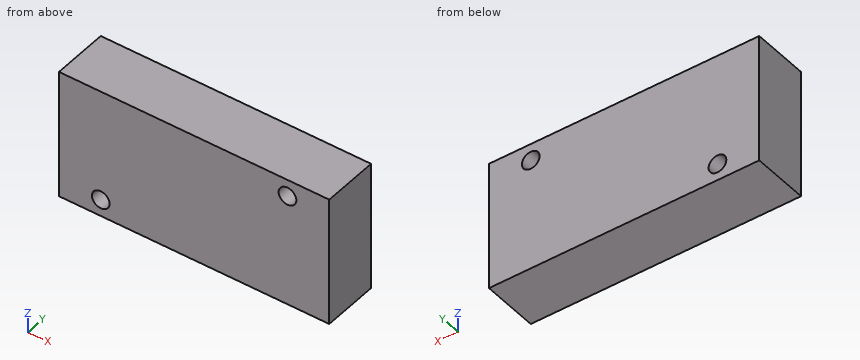
Autodesk Inventor part; units mm, degrees
ref_plane "YZ Plane" through (0, 0, 0) normal (1, 0, 0) x (0, 1, 0)
ref_plane "XZ Plane" through (0, 0, 0) normal (0, 1, 0) x (-1, 0, 0)
ref_plane "XY Plane" through (0, 0, 0) normal (0, 0, 1) x (1, 0, 0)
sketch "Эскиз1" plane through (0, 0, 0) normal (0, 1, 0) x (-1, 0, 0)
  line L0 (24, -11.5) -> (-24, -11.5)
  line L1 (-24, -11.5) -> (-24, 11.5)
  line L2 (-24, 11.5) -> (24, 11.5)
  line L3 (24, 11.5) -> (24, -11.5)
  line L4 (24, -11.5) -> (-24, 11.5) construction
  line L5 (-24, -11.5) -> (24, 11.5) construction
  point P0 (0, 0)
  dimension "d0" = 48
  dimension "d1" = 23
extrude "Выдавливание1" add sketch "Эскиз1" along normal blind 10
sketch "Эскиз2" plane through (0, 10, 0) normal (0, 1, 0) x (1, 0, 0)
  circle A0 centre (16.58, -8.5) radius 1.575
  circle A1 centre (-16.58, 8.5) radius 1.575
  line L0 (24, -11.5) -> (24, 11.5)
  line L1 (-24, -11.5) -> (24, -11.5)
  line L2 (24, 11.5) -> (-24, 11.5)
  line L3 (-24, 11.5) -> (-24, -11.5)
  point P0 (0, 0)
  dimension "d4" = 3.15
  dimension "d5" = 3.15
  dimension "d6" = 40.58
  dimension "d7" = 20
  dimension "d8" = 20
  dimension "d9" = 40.58
extrude "Выдавливание2" cut sketch "Эскиз2" against normal blind 10 contours A0 | A1
properties part number "стабилизатор"
Source: CAD feature listing. Evaluate the final solid. Frame: model axes, mm. Give positions to 0.01 mm unless a question says otherwise; leave off trailing zeros. Write each loop counter-clockwise with the first axis right and the second up, starting at its lowest first coordinate (ties: lowest second). Pieces come first, ordered by that corner, then holes.
1. Material intervals for line 1 along X through (y, z) = (4, 8.5) (3 decimals); line 2 along Z through (x, y) = (-16.58, 5.5) (3 decimals); line 3 along Z through (x, y) = (16.58, 2) (3 decimals), sorted ascending.
2. First-contact query: pin 1 (10 mm diameter, centred on x = 0.5, z = 5.5, fed in from -Y); pin 2 (2.5 mm diameter, centred on x = 16.58, z = 8.5, fed in from -Y). Flat tips, straight axial feed; report the tip coordinate or a pass-through.
3. Section query A-A (x = 16.58). Return the cut outline in (y, z) (3 decimals).
4. Section query B-B (z = 8.5). Return the cut outline in (x, y) (3 decimals), then the cut area to 4 significant figures.
Output values:
1. line 1: x = -24 to 15.005, 18.155 to 24
1. line 2: z = -11.5 to -10.075, -6.925 to 11.5
1. line 3: z = -11.5 to 6.925, 10.075 to 11.5
2. pin 1: stops at y = 0
2. pin 2: passes through
3. outline: (0, -11.5) - (10, -11.5) - (10, 6.925) - (0, 6.925) - close; (0, 10.075) - (10, 10.075) - (10, 11.5) - (0, 11.5) - close
4. outline: (-24, 0) - (15.005, 0) - (15.005, 10) - (-24, 10) - close; (18.155, 0) - (24, 0) - (24, 10) - (18.155, 10) - close
4. area: 448.5 mm2
